from build123d import *

# Parameters (mm, degrees)
SKETCH_W            = 30
SKETCH_H            = 15
PAD_DEPTH           = 3.5
POCKET_DEPTH        = 15.001
LINEARPATTERN_COUNT = 2
LINEARPATTERN_PITCH = 15
SKETCH002_W         = 30
SKETCH002_H         = 15
SKETCH002_W_2       = 28
SKETCH002_H_2       = 13
PAD001_DEPTH        = 4
SKETCH003_W         = 9
SKETCH003_H         = 13
PAD002_DEPTH        = 1
SKETCH004_W         = 2
SKETCH004_H         = 13
PAD003_DEPTH        = 2.5
SKETCH005_W         = 3.6
SKETCH005_H         = 0.9
PAD004_DEPTH        = 3
CHAMFER_SIZE        = 0.5
SKETCH006_W         = 13
SKETCH006_H         = 2.5
POCKET001_DEPTH     = 1
SKETCH007_W         = 8
SKETCH007_H         = 2.5
POCKET002_DEPTH     = 1
SKETCH008_W         = 5
SKETCH008_H         = 1
PAD005_DEPTH        = 0.4
CHAMFER001_SIZE     = 0.39


with BuildPart() as part:
    # Sketch → Pad (new body)
    with BuildSketch(Plane.XY):
        Rectangle(SKETCH_W, SKETCH_H)
    extrude(amount=PAD_DEPTH)

    # Sketch001 (on Face3 of Pad) → Pocket (cut, through all)
    with BuildSketch(Plane.XZ.offset(7.5)):
        with BuildLine():
            Line((-9, 0), (-9, 0.722949))
            ThreePointArc((-9.714159, 2.8), (-9.62774, 1.668412), (-9, 0.722949))
            Line((-9.714159, 2.8), (-5.285841, 2.8))
            ThreePointArc((-6, 0.722949), (-5.37226, 1.668412), (-5.285841, 2.8))
            Line((-6, 0), (-6, 0.722949))
            Line((-9, 0), (-6, 0))
        make_face()
    pocket = extrude(amount=-POCKET_DEPTH, mode=Mode.SUBTRACT)

    # LinearPattern: Pocket ×2
    with Locations(*[(i * LINEARPATTERN_PITCH, 0, 0) for i in range(1, LINEARPATTERN_COUNT)]):
        add(pocket, mode=Mode.SUBTRACT)

    # Sketch002 (on Face16 of LinearPattern) → Pad001 (join)
    with BuildSketch(Plane.XY.offset(3.5)):
        Rectangle(SKETCH002_W, SKETCH002_H)
        Rectangle(SKETCH002_W_2, SKETCH002_H_2, mode=Mode.SUBTRACT)
    extrude(amount=PAD001_DEPTH)

    # Sketch003 (on Face27 of Pad001) → Pad002 (join)
    with BuildSketch(Plane.XY.offset(3.5)):
        Rectangle(SKETCH003_W, SKETCH003_H)
    extrude(amount=PAD002_DEPTH)

    # Sketch004 (on Face27 of Pad002) → Pad003 (join)
    with BuildSketch(Plane.XY.offset(3.5)):
        with Locations((-9.1, 0)):
            Rectangle(SKETCH004_W, SKETCH004_H)
        with Locations((9.1, 0)):
            Rectangle(SKETCH004_W, SKETCH004_H)
    extrude(amount=PAD003_DEPTH)

    # Sketch005 (on Face27 of Pad003) → Pad004 (join)
    with BuildSketch(Plane.XY.offset(3.5)):
        with Locations((-6.3, 6.05)):
            Rectangle(SKETCH005_W, SKETCH005_H)
        with Locations((6.3, 6.05)):
            Rectangle(SKETCH005_W, SKETCH005_H)
        with Locations((-6.3, -6.05)):
            Rectangle(SKETCH005_W, SKETCH005_H)
        with Locations((6.3, -6.05)):
            Rectangle(SKETCH005_W, SKETCH005_H)
    extrude(amount=PAD004_DEPTH)

    # Chamfer
    chamfer_edges = [part.edges().sort_by_distance(p)[0] for p in [
        (-6.3, 5.6, 6.5),
        (6.3, 5.6, 6.5),
        (-6.3, -5.6, 6.5),
        (6.3, -5.6, 6.5),
    ]]
    chamfer(chamfer_edges, length=CHAMFER_SIZE)

    # Sketch006 (on Face35 of Chamfer) → Pocket001 (cut)
    with BuildSketch(Plane(origin=(-15, 0, 0), x_dir=(0, -1, 0), z_dir=(-1, 0, 0))):
        with Locations((0, 6.25)):
            Rectangle(SKETCH006_W, SKETCH006_H)
    extrude(amount=-POCKET001_DEPTH, mode=Mode.SUBTRACT)

    # Sketch007 (on Face29 of Pocket001) → Pocket002 (cut)
    with BuildSketch(Plane.YZ.offset(15)):
        with Locations((0, 6.25)):
            Rectangle(SKETCH007_W, SKETCH007_H)
    extrude(amount=-POCKET002_DEPTH, mode=Mode.SUBTRACT)

    # Sketch008 (on Face21 of Pocket002) → Pad005 (join)
    with BuildSketch(Plane.XZ.offset(-6.5)):
        with Locations((0, 7)):
            Rectangle(SKETCH008_W, SKETCH008_H)
    pad005 = extrude(amount=PAD005_DEPTH)

    # Mirrored: Pad005 across XZ
    add(pad005.mirror(Plane.XZ))

    # Chamfer001
    chamfer001_edges = [part.edges().sort_by_distance(p)[0] for p in [
        (0, -6.1, 7.5),
        (0, 6.1, 7.5),
    ]]
    chamfer(chamfer001_edges, length=CHAMFER001_SIZE)


solid = part.part
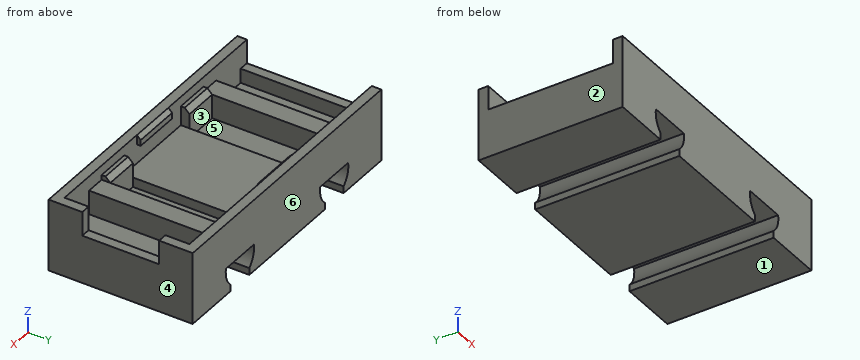
CAD build for the part. Positions are in the model's coordinates, mm. Face numbers are marked on the shaded views. A direction names the side the tool comes from. Round coordinates to 2 decimals unless told otherwise and drop trailing zeros. Write each loop counter-clockwise with the first axis right and the second up, starting at its lowest first coordinate (ties: lowest second). Pieces come first, ordered by that corner, then holes. Notation, with made-up numbers: M -11,1 L 21,1 A20 cw 21,21 Z; hole C 6.25,35 d8. An arc over 180 degrees is marked long. Use a Markdown table: item, result. Add a question column.
1. Drill centre lines: probe 1 along X at (y, z) = (-5, 3.75); probe 2 along Y at (x, z) = (-13.5, 4); probe 3 along X at (y, z) = (6.25, 2.75). Where is each one in solid material? Low to high.
2. 3-axis set-ups, long thin cutter, end or side, ignore diameter. For the marked faces 5 and 6: which of +Z, -Z, +X, -X, +Y, -Y reach the whole face in a straight line?
3. Pull direction X, two halves, no side cores. Call the marked faces 1, 2, 3 and 4: released by +X, released by -X, zero draft, split by the parting line, or undercut.
4. Slice it at C-C on z = 5.5. Give the cut face in (x, y).
5. Flat gauge pins, fed straight in: P1, Ø2.5, axis at x = 2, y = 2, coming from the +Z side; P2, Ø1.5, axis at y = 1.5, z = 6, coming from the -X side; P3, Ø1.8, axis at x = 6.5, y = 1, coming from the +Z side. Where does each tip first touch, or does it go through?
6. Slice it at A-A on z = 2. Give the cut face in (x, y).
7. Slice it at D-D on x = 11.75. Give the cut face in (y, z).
Reply:
| question | item | result |
|---|---|---|
| 1 | probe 1 | x = -15 to -14, -10.1 to -8.1, -4.5 to 4.5, 8.1 to 10.1, 14 to 15 |
| 1 | probe 2 | y = -7.5 to -6.5, 6.5 to 7.5 |
| 1 | probe 3 | x = -15 to -9.72, -5.28 to 5.28, 9.72 to 15 |
| 2 | face 5 | +Z |
| 2 | face 6 | +Z, -Z, +X, -X, +Y |
| 3 | face 1 | zero draft |
| 3 | face 2 | released by -X |
| 3 | face 3 | undercut |
| 3 | face 4 | released by +X |
| 4 | outline | M -15,-7.5 L 15,-7.5 L 15,-4 L 14,-4 L 14,-6.5 L 10.1,-6.5 L 10.1,6.5 L 14,6.5 L 14,4 L 15,4 L 15,7.5 L -15,7.5 L -15,6.5 L -10.1,6.5 L -10.1,-6.5 L -15,-6.5 Z; hole M -8.1,-5.6 L -4.5,-5.6 L -4.5,-6.5 L 4.5,-6.5 L 4.5,-5.6 L 8.1,-5.6 L 8.1,5.6 L 4.5,5.6 L 4.5,6.5 L -4.5,6.5 L -4.5,5.6 L -8.1,5.6 Z |
| 5 | P1 | stops at z = 4.5 |
| 5 | P2 | stops at x = -10.1 |
| 5 | P3 | stops at z = 3.5 |
| 6 | outline | M -15,-7.5 L -9.71,-7.5 L -9.71,7.5 L -15,7.5 Z; M -5.29,-7.5 L 5.29,-7.5 L 5.29,7.5 L -5.29,7.5 Z; M 9.71,-7.5 L 15,-7.5 L 15,7.5 L 9.71,7.5 Z |
| 7 | outline | M -7.5,0 L 7.5,0 L 7.5,7.5 L 6.5,7.5 L 6.5,3.5 L -6.5,3.5 L -6.5,7.5 L -7.5,7.5 Z |
